```python
from build123d import *

# Parameters (mm, degrees)
F0_R     = 50
F1_DEPTH = 100
F2_W     = 20
F2_H     = 30
F3_DEPTH = 55


with BuildPart() as f1:
    # F0 (on Top) → F1 (new body)
    with BuildSketch(Plane.XY):
        Circle(F0_R)
    extrude(amount=F1_DEPTH)

    # F2 (on Front) → F3 (join)
    with BuildSketch(Plane.XZ):
        with Locations((0, 50.83777)):
            Rectangle(F2_W, F2_H)
    extrude(amount=F3_DEPTH)


solid = f1.part
```
Source: CAD feature listing. Evaluate the final solid. Frame: model axes, mm. A direction names the side the tool comes from. Coordinates: 2 decimals unless noted, no trailing zeros. Loops run counter-clockwise (first coordinate to the right, second up) from the corner with the lowest first, then second, coordinate; pieces in that order, holes last. Notation, with made-up numbers: (64.5, 40.25) -> (86.5, 40.25) arc R15 cw to (86.5, 65.25) -> close; hole circle Ø7 at (30.25, 53). An arc over 180 degrees is marked (long way). One line per item, written item: value. Start each with the question number.
Q1. Section query B-B, the plane z = 16. Return the cut outline in (x, y).
Q2. Set-up query: faces 1 (the face through (-10, -52, 51)), 2 (the face through (10, -52, 51)), 3 (the face through (-1, 1, 100)). Return all of +Z, -Z, +X, -X, +Y, -Y with unobstructed straight access to the full face (end or side cutting, diameter ignored); none if empty.
Q3. Section query A-A, the plane x = 0. Return the cut outline in (y, z).
Q4. Line query: line 1 along Y through (x, z) = (21, 56); line 2 along Y through (x, z) = (44, 10); line 3 along X through (y, z) = (-25, 64). Output: solid intervals per line, ascending.
Q5. Section query D-D, the plane x = 14. Return the cut outline in (y, z), and give its area (3 significant figures).
Q6. Contact query for flat-ended pins moving along their axis: P1, Ø3, axis at y = -51, z = 51, coming from the +X side; P2, Ø3, axis at x = -1.5, y = -52.5, coming from the +Z side; P3, Ø2, axis at y = 20.5, z = 26.5, coming from the -X side. Output: stop coordinate, or through.
Q7. Section query C-C, the plane y = 40.5. Return the cut outline in (x, z), and give its area (3 significant figures).
Results:
1. outline: circle Ø100 at (0, 0)
2. face 1: +Z, -Z, -X, -Y
2. face 2: +Z, -Z, +X, -Y
2. face 3: +Z, +X, -X, +Y, -Y
3. outline: (-55, 35.84) -> (-50, 35.84) -> (-50, 0) -> (50, 0) -> (50, 100) -> (-50, 100) -> (-50, 65.84) -> (-55, 65.84) -> close
4. line 1: -45.38 to 45.38
4. line 2: -23.75 to 23.75
4. line 3: -43.3 to 43.3
5. outline: (-48, 0) -> (48, 0) -> (48, 100) -> (-48, 100) -> close
5. area: 9,600 mm^2
6. P1: x = 10
6. P2: z = 65.84
6. P3: x = -46.04
7. outline: (-29.32, 0) -> (29.32, 0) -> (29.32, 100) -> (-29.32, 100) -> close
7. area: 5,860 mm^2
